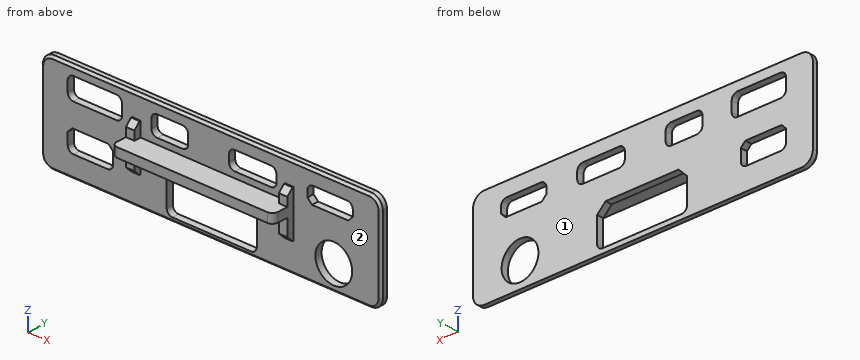
from build123d import *

# Parameters (mm, degrees)
SKETCH_1_W          = 60
SKETCH_1_H          = 17
EXTRUDE_1_DEPTH     = 1.2
CUT_EXTRUDE_1_REACH = 33.204
SKETCH_4_R          = 3.25
SKETCH_4_W          = 8
SKETCH_4_H          = 3.8
SKETCH_4_W_2        = 15.9
SKETCH_4_H_2        = 6.8
SKETCH_4_H_3        = 2.9
SKETCH_4_W_3        = 8.4
SKETCH_4_H_4        = 3.2
SKETCH_4_W_4        = 6.5
SKETCH_4_H_5        = 3.5
SKETCH_4_W_5        = 9.6
FILLET_2_R          = 1
CHAMFER_1_SIZE      = 0.8
SKETCH_5_W          = 1.5
SKETCH_5_H          = 8
EXTRUDE_2_DEPTH     = 1.2
SKETCH_6_W          = 28.5
SKETCH_6_H          = 1.6
EXTRUDE_3_DEPTH     = 4
FILLET_3_R          = 1
CHAMFER_2_SIZE      = 1
FILLET_4_R          = 2
CHAMFER_5_SIZE      = 0.4
CHAMFER_6_SIZE      = 1.5


with BuildPart() as part:
    # 草图1 → 凸台-拉伸1 (new body)
    with BuildSketch(Plane(origin=(0, 0, 0), x_dir=(1, 0, 0), z_dir=(0, 1, 0))):
        Rectangle(SKETCH_1_W, SKETCH_1_H)
    extrude(amount=EXTRUDE_1_DEPTH)

    # 草图4 → 切除-拉伸1 (cut, up to next)
    with BuildSketch(Plane(origin=(0, 1.2, 0), x_dir=(1, 0, 0), z_dir=(0, 1, 0)), mode=Mode.PRIVATE) as cut_extrude_1_sk1:
        with Locations(Location((21.7, 4.2, 0), (0, 0, 270))):
            Circle(SKETCH_4_R)
    cut_extrude_1_tool1 = extrude(cut_extrude_1_sk1.sketch, amount=-CUT_EXTRUDE_1_REACH, mode=Mode.PRIVATE) & part.part
    # 草图4 → 切除-拉伸1 (cut, up to next)
    with BuildSketch(Plane(origin=(0, 1.2, 0), x_dir=(1, 0, 0), z_dir=(0, 1, 0)), mode=Mode.PRIVATE) as cut_extrude_1_sk2:
        with Locations((-21.271722325, 2.8)):
            Rectangle(SKETCH_4_W, SKETCH_4_H)
    cut_extrude_1_tool2 = extrude(cut_extrude_1_sk2.sketch, amount=-CUT_EXTRUDE_1_REACH, mode=Mode.PRIVATE) & part.part
    # 草图4 → 切除-拉伸1 (cut, up to next)
    with BuildSketch(Plane(origin=(0, 1.2, 0), x_dir=(1, 0, 0), z_dir=(0, 1, 0)), mode=Mode.PRIVATE) as cut_extrude_1_sk3:
        with Locations((0.15, 4.3)):
            Rectangle(SKETCH_4_W_2, SKETCH_4_H_2)
    cut_extrude_1_tool3 = extrude(cut_extrude_1_sk3.sketch, amount=-CUT_EXTRUDE_1_REACH, mode=Mode.PRIVATE) & part.part
    # 草图4 → 切除-拉伸1 (cut, up to next)
    with BuildSketch(Plane(origin=(0, 1.2, 0), x_dir=(1, 0, 0), z_dir=(0, 1, 0)), mode=Mode.PRIVATE) as cut_extrude_1_sk4:
        with Locations((21.05, -4.584803861)):
            Rectangle(SKETCH_4_W, SKETCH_4_H_3)
    cut_extrude_1_tool4 = extrude(cut_extrude_1_sk4.sketch, amount=-CUT_EXTRUDE_1_REACH, mode=Mode.PRIVATE) & part.part
    # 草图4 → 切除-拉伸1 (cut, up to next)
    with BuildSketch(Plane(origin=(0, 1.2, 0), x_dir=(1, 0, 0), z_dir=(0, 1, 0)), mode=Mode.PRIVATE) as cut_extrude_1_sk5:
        with Locations((7.4, -4.734803861)):
            Rectangle(SKETCH_4_W_3, SKETCH_4_H_4)
    cut_extrude_1_tool5 = extrude(cut_extrude_1_sk5.sketch, amount=-CUT_EXTRUDE_1_REACH, mode=Mode.PRIVATE) & part.part
    # 草图4 → 切除-拉伸1 (cut, up to next)
    with BuildSketch(Plane(origin=(0, 1.2, 0), x_dir=(1, 0, 0), z_dir=(0, 1, 0)), mode=Mode.PRIVATE) as cut_extrude_1_sk6:
        with Locations((-7.25, -4.884803861)):
            Rectangle(SKETCH_4_W_4, SKETCH_4_H_5)
    cut_extrude_1_tool6 = extrude(cut_extrude_1_sk6.sketch, amount=-CUT_EXTRUDE_1_REACH, mode=Mode.PRIVATE) & part.part
    # 草图4 → 切除-拉伸1 (cut, up to next)
    with BuildSketch(Plane(origin=(0, 1.2, 0), x_dir=(1, 0, 0), z_dir=(0, 1, 0)), mode=Mode.PRIVATE) as cut_extrude_1_sk7:
        with Locations((-20.471722325, -5.034803861)):
            Rectangle(SKETCH_4_W_5, SKETCH_4_H)
    cut_extrude_1_tool7 = extrude(cut_extrude_1_sk7.sketch, amount=-CUT_EXTRUDE_1_REACH, mode=Mode.PRIVATE) & part.part
    add(cut_extrude_1_tool1.solids().sort_by_distance((21.7, 1.2, -4.2))[0], mode=Mode.SUBTRACT)
    add(cut_extrude_1_tool2.solids().sort_by_distance((-21.271722, 1.2, -2.8))[0], mode=Mode.SUBTRACT)
    add(cut_extrude_1_tool3.solids().sort_by_distance((0.15, 1.2, -4.3))[0], mode=Mode.SUBTRACT)
    add(cut_extrude_1_tool4.solids().sort_by_distance((21.05, 1.2, 4.584804))[0], mode=Mode.SUBTRACT)
    add(cut_extrude_1_tool5.solids().sort_by_distance((7.4, 1.2, 4.734804))[0], mode=Mode.SUBTRACT)
    add(cut_extrude_1_tool6.solids().sort_by_distance((-7.25, 1.2, 4.884804))[0], mode=Mode.SUBTRACT)
    add(cut_extrude_1_tool7.solids().sort_by_distance((-20.471722, 1.2, 5.034804))[0], mode=Mode.SUBTRACT)

    # 圆角2
    fillet_2_edges = [part.edges().sort_by_distance(p)[0] for p in [
        (-10.5, 0.6, 6.634803861),
        (-10.5, 0.6, 3.134803861),
        (-4, 0.6, 3.134803861),
        (-4, 0.6, 6.634803861),
        (3.2, 0.6, 6.334803861),
        (3.2, 0.6, 3.134803861),
        (11.6, 0.6, 3.134803861),
        (11.6, 0.6, 6.334803861),
        (17.05, 0.6, 6.034803861),
        (25.05, 0.6, 6.034803861),
        (-7.8, 0.6, -7.7),
        (8.1, 0.6, -7.7),
        (-25.271722325, 0.6, 6.934803861),
        (-25.271722325, 0.6, 3.134803861),
        (-15.671722325, 0.6, 3.134803861),
        (-15.671722325, 0.6, 6.934803861),
        (-25.271722325, 0.6, -4.7),
        (-17.271722325, 0.6, -4.7),
    ]]
    fillet(fillet_2_edges, radius=FILLET_2_R)

    # 倒角1
    chamfer_1_edges = [part.edges().sort_by_distance(p)[0] for p in [
        (17.05, 0.6, 3.134803861),
        (25.05, 0.6, 3.134803861),
        (-25.271722325, 0.6, -0.9),
        (-17.271722325, 0.6, -0.9),
    ]]
    chamfer(chamfer_1_edges, length=CHAMFER_1_SIZE)

    # 草图5 → 凸台-拉伸2 (add)
    with BuildSketch(Plane.XZ):
        with Locations((-13.15891381, 0.61681071)):
            Rectangle(SKETCH_5_W, SKETCH_5_H)
        with Locations((13.84108619, 0.61681071)):
            Rectangle(SKETCH_5_W, SKETCH_5_H)
    extrude(amount=EXTRUDE_2_DEPTH)

    # 草图6 → 凸台-拉伸3 (add)
    with BuildSketch(Plane.XZ):
        with Locations((0.34108619, 1.3)):
            Rectangle(SKETCH_6_W, SKETCH_6_H)
    extrude(amount=EXTRUDE_3_DEPTH)

    # 圆角3
    fillet_3_edges = [part.edges().sort_by_distance(p)[0] for p in [
        (-13.90891381, -4, 1.3),
        (14.59108619, -4, 1.3),
    ]]
    fillet(fillet_3_edges, radius=FILLET_3_R)

    # 倒角2
    chamfer_2_edges = [part.edges().sort_by_distance(p)[0] for p in [
        (-13.15891381, -1.2, -3.38318929),
        (-13.15891381, -1.2, 4.61681071),
        (13.84108619, -1.2, -3.38318929),
        (13.84108619, -1.2, 4.61681071),
    ]]
    chamfer(chamfer_2_edges, length=CHAMFER_2_SIZE)

    # 圆角4
    fillet_4_edges = [part.edges().sort_by_distance(p)[0] for p in [
        (30, 0.6, 8.5),
        (-30, 0.6, 8.5),
        (-30, 0.6, -8.5),
        (30, 0.6, -8.5),
    ]]
    fillet(fillet_4_edges, radius=FILLET_4_R)

    # 倒角5
    chamfer_5_edges = [part.edges().sort_by_distance(p)[0] for p in [
        (30, 0, 0),
        (0, 0, 8.5),
        (-30, 0, 0),
        (0, 0, -8.5),
        (-29.414213562, 0, -7.914213562),
        (-29.414213562, 0, 7.914213562),
        (29.414213562, 0, -7.914213562),
        (29.414213562, 0, 7.914213562),
    ]]
    chamfer(chamfer_5_edges, length=CHAMFER_5_SIZE)

    # 倒角6
    chamfer_6_edges = [part.edges().sort_by_distance(p)[0] for p in [
        (-7.8, 0.6, -0.9),
        (8.1, 0.6, -0.9),
    ]]
    chamfer(chamfer_6_edges, length=CHAMFER_6_SIZE)


solid = part.part
The model under review builds one solid part; all positions refer to its coordinate system, in mm. Face numbers are marked on the shaded views. Round coordinates to 2 decimals unless told otherwise and drop trailing zeros. Loops run counter-clockwise (first coordinate to the right, second up) from the corner with the lowest first, then second, coordinate; pieces in that order, holes last. Notation, with made-up numbers: M 33,4 L 47,4 A28 cw 47,40 Z; hole C 31,6 d3. An arc over 180 degrees is marked long. Answer as a JSON object with one key per item and string values.
Item 1: Clearance check with flat-ended pins moving along their axes: P1, Ø0.8, axis at x = 14, z = 3, coming from the -Y side; P2, Ø1.5, axis at x = 17, z = 4.5, coming from the -Y side; P3, Ø2, axis at x = 21, y = -2, coming from the -Z side; P4, Ø2, axis at x = -6.5, y = -2.5, coming from the -Z side. State where each tip first meets the part, or that it passes through.
Check sheet entries:
{"P1": "y = -1.2", "P2": "y = 0", "P3": "through", "P4": "z = 0.5"}
Item 2: The part is to be moulded in two halves that separate along X. For the marked faces 1 and 2, say which applies: +X half, -X half, draft (parallel to the pull), parting line (faces both ways), or undercut.
Check sheet entries:
{"face 1": "draft", "face 2": "undercut"}
Item 3: We need section A-A, the plane x = 2. State the section outline as (y, z) points, and give its area (3 significant figures).
Check sheet entries:
{"outline": "M -4,0.5 L 0,0.5 L 0,-0.9 L 1.2,-0.9 L 1.2,8.5 L 0.4,8.5 L 0,8.1 L 0,2.1 L -4,2.1 Z; M 0,-8.1 L 0.4,-8.5 L 1.2,-8.5 L 1.2,-7.7 L 0,-7.7 Z", "area": "18.5 mm2"}
Item 4: We need section B-B, the plane x = 21.7. State the section outline as (y, z) points, and give its area (3 significant figures).
Check sheet entries:
{"outline": "M 0,-8.1 L 0.4,-8.5 L 1.2,-8.5 L 1.2,-7.45 L 0,-7.45 Z; M 0,-0.95 L 1.2,-0.95 L 1.2,3.13 L 0,3.13 Z; M 0,6.03 L 1.2,6.03 L 1.2,8.5 L 0.4,8.5 L 0,8.1 Z", "area": "8.96 mm2"}
Item 5: For line 1 along Z through (x, y) = (-5, 0.65); line 2 along X through (y, z) = (0.35, -4.2); line 3 along X through (y, z) = (0.7, 6.5), list the stretches that pass through material, from the lowest coordinate up.
Check sheet entries:
{"line 1": "-8.5 to -7.7, -0.9 to 3.13, 6.63 to 8.5", "line 2": "-29.95 to -25.14, -17.41 to -7.8, 8.1 to 18.45, 24.95 to 29.95", "line 3": "-30 to -25.1, -15.85 to -10, -4.5 to 30"}
